```python
from build123d import *

# Parameters (mm, degrees)
F1_DEPTH  = 25.4
F3_DEPTH  = 25.4
F5_DEPTH  = 25.4
F7_DEPTH  = 25.4
F8_R      = 3.725598
F8_R_2    = 3.542164
F9_DEPTH  = 25.4
F10_R     = 4.455747
F11_DEPTH = 25.4


with BuildPart() as f1:
    # F0 (on Front) → F1 (new body)
    with BuildSketch(Plane.XZ):
        Polygon((-32.395763, 12.7), (-32.395763, 0), (43.804237, 0), (43.804237, 12.7), (18.404237, 12.7), (18.404237, 36.485594), (-6.995763, 36.485594), (-6.995763, 12.7), align=None)
    extrude(amount=F1_DEPTH)

    # F2 (on face) → F3 (cut)
    with BuildSketch(Plane(origin=(-6.995763, 0, 0), x_dir=(0, -1, 0), z_dir=(-1, 0, 0))):
        with BuildLine():
            ThreePointArc((0, 28.142773), (12.583745, 36.02061), (25.4, 28.526975))
            Line((25.4, 28.526975), (25.4, 36.485594))
            Line((25.4, 36.485594), (0, 36.485594))
            Line((0, 36.485594), (0, 28.142773))
        make_face()
    extrude(amount=-F3_DEPTH, mode=Mode.SUBTRACT)

    # F4 (on face) → F5 (cut)
    with BuildSketch(Plane.XY.offset(12.7)):
        with BuildLine():
            ThreePointArc((-23.340253, -25.4), (-31.730093, -12.434566), (-22.571849, 0))
            Line((-22.571849, 0), (-32.395763, 0))
            Line((-32.395763, 0), (-32.395763, -25.4))
            Line((-32.395763, -25.4), (-23.340253, -25.4))
        make_face()
    extrude(amount=-F5_DEPTH, mode=Mode.SUBTRACT)

    # F6 (on face) → F7 (cut)
    with BuildSketch(Plane.XY.offset(12.7)):
        with BuildLine():
            ThreePointArc((36.787312, 0), (43.280053, -12.604697), (37.171513, -25.4))
            Line((37.171513, -25.4), (43.804237, -25.4))
            Line((43.804237, -25.4), (43.804237, 0))
            Line((43.804237, 0), (36.787312, 0))
        make_face()
    extrude(amount=-F7_DEPTH, mode=Mode.SUBTRACT)

    # F8 (on face) → F9 (cut)
    with BuildSketch(Plane.XY.offset(12.7)):
        with Locations((-18.151755, -12.84534)):
            Circle(F8_R)
        with Locations((30.063784, -13.158907)):
            Circle(F8_R_2)
    extrude(amount=-F9_DEPTH, mode=Mode.SUBTRACT)

    # F10 (on face) → F11 (cut)
    with BuildSketch(Plane(origin=(-6.995763, 0, 0), x_dir=(0, -1, 0), z_dir=(-1, 0, 0))):
        with Locations((12.582604, 25.837563)):
            Circle(F10_R)
    extrude(amount=-F11_DEPTH, mode=Mode.SUBTRACT)


solid = f1.part
```
The model under review builds one solid part; all positions refer to its coordinate system, in mm. A direction names the side the tool comes from. Give positions to 0.01 mm unless a question says otherwise; leave off trailing zeros. Loops run counter-clockwise (first coordinate to the right, second up) from the corner with the lowest first, then second, coordinate; pieces in that order, holes last. Notation, with made-up numbers: (-25, -3) - (28, -3) arc R23 cw to (28, 6) - close; hole circle Ø8 at (43.25, 40.25). An arc over 180 degrees is marked (long way). Answer as a JSON object with one key per item and string values.
Q1. Mouldability with a two-part tool opening along Z and no side actions: class faces 1 (the flat face through (5, -13, 0)), 2 (the cylindrical face through (5.526, -11.617, 21.488)), 3 (the flat face through (-6.996, -15.3, 21.9)) as +Z half, -Z half, draft (parallel to the pull), parting line (faces both ways), or undercut.
Worked out:
{"face 1": "-Z half", "face 2": "undercut", "face 3": "draft"}
Q2. Add section D-D on x = 11.5. State the section outline as (y, z) points.
Worked out:
{"outline": "(-25.4, 0) - (0, 0) - (0, 28.14) arc R14.34 ccw to (-25.4, 28.53) - close; hole circle Ø8.91 at (-12.58, 25.84)"}
Q3. Insertion check: pin 1 (11.5 mm diameter, centred on y = -6.5, z = 25.5, fed in from +X); pin 2 (5 mm diameter, centred on y = -10, z = 12, fed in from -X); pin 3 (2 mm diameter, centred on y = -7.5, z = 6.5, fed in from +X); pin 4 (6 mm diameter, centred on y = -16, z = 7, fed in from +X). Each pin has a flat end and moves straight along its axis. Give the tip position at first contact, or say it passes through.
Worked out:
{"pin 1": "stops at x = 18.4", "pin 2": "stops at x = -31.73", "pin 3": "stops at x = 42.68", "pin 4": "stops at x = 43.28"}
Q4. To check wall thickness, follow line 1 along X through (y, z) = (-15.75, 3); line 2 along X through (y, z) = (-21.25, 19.5); line 3 along Z through (x, y) = (30, -18.25). State the ranges of each line that lie inside material, in increasing order.
Worked out:
{"line 1": "x = -31.42 to -20.48, -15.82 to 27.65, 32.48 to 43.02", "line 2": "x = -7 to 18.4", "line 3": "z = 0 to 12.7"}
Q5. Add section C-C on z = 18. State the section outline as (x, y) points, plus the area to 3 significant figures.
Worked out:
{"outline": "(-7, -25.4) - (18.4, -25.4) - (18.4, 0) - (-7, 0) - close", "area": "645 mm^2"}
Q6. Add section A-A on x = -15.5. State the section outline as (y, z) points.
Worked out:
{"outline": "(-25.4, 0) - (-15.46, 0) - (-15.46, 12.7) - (-25.4, 12.7) - close; (-10.23, 0) - (0, 0) - (0, 12.7) - (-10.23, 12.7) - close"}
Q7. For faces 4 (the flat face through (28, -10, 12.7)), 5 (the flat face through (-22, -15, 12.7)), 6 (the cylindrical face through (6, -12, 36)), list the 3-axis set-ups (+Z, -Z, +X, -X, +Y, -Y) from which the entire face can be reached by the end or side of a thin tool; tool diameter is ignored.
Worked out:
{"face 4": "+Z, +X, +Y, -Y", "face 5": "+Z, -X, +Y, -Y", "face 6": "+Z, +X, -X"}
Q8. Add section B-B on y = -15.75. State the section outline as (x, z) points.
Worked out:
{"outline": "(-31.42, 0) - (-20.48, 0) - (-20.48, 12.7) - (-31.42, 12.7) - close; (-15.82, 0) - (27.65, 0) - (27.65, 12.7) - (18.4, 12.7) - (18.4, 22.7) - (-7, 22.7) - (-7, 12.7) - (-15.82, 12.7) - close; (-7, 28.97) - (18.4, 28.97) - (18.4, 35.72) - (-7, 35.72) - close; (32.48, 0) - (43.02, 0) - (43.02, 12.7) - (32.48, 12.7) - close"}
